Autodesk Inventor part; units mm, degrees
ref_plane "YZ Plane" through (0, 0, 0) normal (1, 0, 0) x (0, 1, 0)
ref_plane "XZ Plane" through (0, 0, 0) normal (0, 1, 0) x (-1, 0, 0)
ref_plane "XY Plane" through (0, 0, 0) normal (0, 0, 1) x (1, 0, 0)
sketch "Sketch1" plane through (0, 0, 0) normal (0, 0, 1) x (1, 0, 0)
  circle A0 centre (0, 0) radius 10
  line L0 (0, 10) -> (0, 9)
  line L1 (-7.116, 7.0259) -> (7.116, 7.0259)
  line L2 (7.116, -7.0259) -> (-7.116, -7.0259)
  dimension "d0" = 20
  dimension "d7" = 14.0518
extrude "Extrusion1" add sketch "Sketch1" against normal blind 27 contours A0 L2 L1
sketch "Sketch2" plane through (0, 0, -27) normal (0, 0, -1) x (0, -1, 0)
  circle A0 centre (0, 0) radius 1
  dimension "d4" = 2
extrude "Extrusion2" add sketch "Sketch2" along normal blind 10
properties part number "motor 12v"
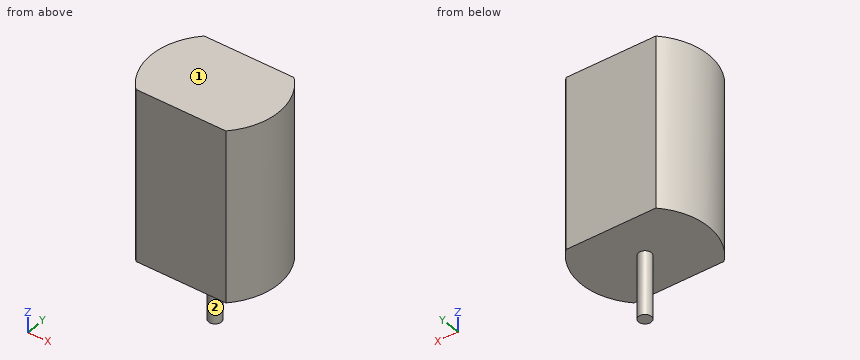
Model file for the job. Use its own axes, mm. Face numbers are marked on the shaded views. A direction names the side the tool comes from. Round coordinates to 2 decimals unless told otherwise and drop trailing zeros. Loops run counter-clockwise (first coordinate to the right, second up) from the corner with the lowest first, then second, coordinate; pieces in that order, holes last. Notation, with made-up numbers: (-17, 42) - (36, 42) arc R9 ccw to (36, 50) - close; hole circle Ø8 at (22, 86.5). An arc over 180 degrees is marked (long way). Write each question's results on one line, items separated by ' | '.
(1) Wall check: L1, parallel to Z at x = -8.75, y = -0.5; L2, parallel to X at y = -0.25, z = -4.5; L3, parallel to X at y = 2, z = -4. Give the ranges that are in metal, low to high.
Answer below:
L1: z = -27 to 0 | L2: x = -10 to 10 | L3: x = -9.8 to 9.8
(2) Saw through at D-D, the plane x = -5. List the corners of the cut face in (y, z), then the cut area to 3 significant figures.
Answer below:
outline: (-7.03, -27) - (7.03, -27) - (7.03, 0) - (-7.03, 0) - close | area: 379 mm^2
(3) Pin check, flat tips, straight feed: pin 1 (3 mm diameter, centred on x = -5.5, y = 0.5, fed in from -Z); pin 2 (1 mm diameter, centred on y = -1, z = -21.5, fed in from -X). Stop position of each tip, or through.
Answer below:
pin 1: stops at z = -27 | pin 2: stops at x = -9.99
(4) Saw through at C-C, the plane z = -28. List the corners of the cut face in (x, y), then the cut area to 3 significant figures.
Answer below:
outline: circle Ø2 at (0, 0) | area: 3.14 mm^2
(5) 3-axis set-ups, long thin cutter, end or side, ignore diameter. For the marked faces 1 and 2: which of +Z, -Z, +X, -X, +Y, -Y reach the whole face in a straight line?
Answer below:
face 1: +Z, +X, -X, +Y, -Y | face 2: -Z
(6) Saw through at B-B, the plane y = 0. List the corners of the cut face in (x, z).
Answer below:
outline: (-10, -27) - (-1, -27) - (-1, -37) - (1, -37) - (1, -27) - (10, -27) - (10, 0) - (-10, 0) - close
(7) Saw through at A-A, the plane x = 0. List the corners of the cut face in (y, z), then the cut area to 3 significant figures.
Answer below:
outline: (-7.03, -27) - (-1, -27) - (-1, -37) - (1, -37) - (1, -27) - (7.03, -27) - (7.03, 0) - (-7.03, 0) - close | area: 399 mm^2
